Could you check a few things on this model? Use its own coordinates, in mm. A direction names the side the tool comes from. Give positions to 0.01 mm unless a question says otherwise; leave off trailing zeros. Loops run counter-clockwise (first coordinate to the right, second up) from the corner with the lowest first, then second, coordinate; pieces in that order, holes last. Notation, with made-up numbers: M 75.5,86.5 L 115.5,86.5 A20 ccw 115.5,119.5 Z; hole C 17,67.25 d6. An arc over 180 degrees is marked long. Write each question's results on one line, items separated by ' | '. Start each with the question number.
Autodesk Inventor part; units mm, degrees
ref_plane "YZ Plane" through (0, 0, 0) normal (1, 0, 0) x (0, 1, 0)
ref_plane "XZ Plane" through (0, 0, 0) normal (0, 1, 0) x (-1, 0, 0)
ref_plane "XY Plane" through (0, 0, 0) normal (0, 0, 1) x (1, 0, 0)
sketch "Эскиз1" plane through (0, 0, 0) normal (1, 0, 0) x (0, 1, 0)
  line L0 (-0.0944, -29.3854) -> (-9.0944, -29.3854)
  line L1 (-9.0944, -29.3854) -> (-9.0944, -27.3854)
  line L2 (-9.0944, -27.3854) -> (-7.0944, -27.3854)
  line L3 (-7.0944, -27.3854) -> (-7.0944, -17.3854)
  line L4 (-7.0944, -17.3854) -> (-0.0944, -17.3854)
  line L5 (-0.0944, -17.3854) -> (-0.0944, -19.3854)
  line L6 (-0.0944, -19.3854) -> (-4.0944, -19.3854)
  line L7 (-4.0944, -19.3854) -> (-4.0944, -20.8854)
  line L8 (-4.0944, -20.8854) -> (-3.0944, -20.8854)
  line L9 (-3.0944, -20.8854) -> (-3.0944, -29.3854)
  line L10 (-0.0944, -15.3854) -> (-0.0944, -31.3854)
  point P0 (0, 0)
  point P1 (-105.6045, -1.7251)
revolve "Вращение1" add sketch "Эскиз1" angle 360 about axis through (0, -0.0944, -15.3854) along (0, 0, -1) contours L0 L1 L2 L3 L4 L5 L6 L7 L8 L9
equation "\"Радиус_гибки\" = Толщина"
equation "\"Ширина_просечки\" = Толщина"
equation "\"Глубина_просечки\" = 0.5 * Толщина"
equation "\"Размер_просечки\" = 4 * Толщина"
equation "\"Мин_остаток\" = 2 * Толщина"
equation "\"Радиус_перехода\" = Радиус_гибки"
equation "\"Радиус_Якоби\" = Радиус_гибки"
equation "\"Размер_зазора\" = Толщина"
1) If we section it at D-D on x = 4.5: Write out the boundary of the cut face in (y, z), plus the area to 3 significant figures.
2) Which directions (+Z, -Z, +X, -X, +Y, -Y) give clear straight access to the entire face, cutting with the end or side of a thin tool? Please do faces 1 (the face through (8.923, 1.077, -28.371)), 2 (the face through (1.825, 2.286, -25.195)), 3 (the face through (3.9, 0.8, -20.1)).
3) If we section it at A-A on x = 0: Write out the boundary of the cut face in (y, z).
4) Thinking about a two-plate mould opening in X: for faces 4 (the face through (7.3, -0.1, -27.385)), 5 (the face through (-6.21, -3.324, -22.315)), 6 (the face through (-3, -2, -20.885)), which applies, pulls with the +X half, pulls with the -X half, needs draft (parallel to the pull), parting line crosses it, or undercut?
5) I'm going to push flat-ended pins straight in: P1, Ø2, axis at x = 6.5, z = -21.5, coming from the -Y side; P2, Ø2, axis at x = -0.5, z = -19.5, coming from the -Y side; P3, Ø1, axis at x = -3.5, z = -20.5, coming from the +Y side; P4, Ø9, axis at x = 1, y = -1.5, coming from the -Z side. Where does each tip first touch, or does it pass through?
6) If we section it at C-C on y = -0.5: Write out the boundary of the cut face in (x, z), plus the area to 3 significant figures.
7) Please list where these lines run through material, in increasing order: line 1 (Y direction, x = 0, z = -20.05); line 2 (Y direction, x = 2, z = -22.75); line 3 (Z direction, x = 7.25, y = 1.25). Write a range as from..to.
8) If we section it at B-B on z = -23.25: Write out the boundary of the cut face in (x, y).
Calculated:
1) outline: M -7.89,-29.39 L 7.7,-29.39 L 7.7,-27.39 L 5.27,-27.39 L 5.27,-17.39 L -5.46,-17.39 L -5.46,-27.39 L -7.89,-27.39 Z | area: 138 mm2
2) face 1: +Z, -Z | face 2: -Z | face 3: none
3) outline: M -9.09,-29.39 L -3.09,-29.39 L -3.09,-20.89 L -4.09,-20.89 L -4.09,-19.39 L 3.91,-19.39 L 3.91,-20.89 L 2.91,-20.89 L 2.91,-29.39 L 8.91,-29.39 L 8.91,-27.39 L 6.91,-27.39 L 6.91,-17.39 L -7.09,-17.39 L -7.09,-27.39 L -9.09,-27.39 Z
4) face 4: needs draft | face 5: parting line crosses it | face 6: undercut
5) P1: stops at y = -4.42 | P2: stops at y = -7.09 | P3: stops at y = 6.23 | P4: stops at z = -29.39
6) outline: M -8.99,-29.39 L -2.97,-29.39 L -2.97,-20.89 L -3.98,-20.89 L -3.98,-19.39 L 3.98,-19.39 L 3.98,-20.89 L 2.97,-20.89 L 2.97,-29.39 L 8.99,-29.39 L 8.99,-27.39 L 6.99,-27.39 L 6.99,-17.39 L -6.99,-17.39 L -6.99,-27.39 L -8.99,-27.39 Z | area: 113 mm2
7) line 1: y = -7.09..-4.09, 3.91..6.91 | line 2: y = -6.8..-2.33, 2.14..6.61 | line 3: z = -29.39..-27.39
8) outline: C 0,-0.09 d14; hole C 0,-0.09 d6
